```python
from build123d import *

# Parameters (mm, degrees)
BOSS_EXTRUDE1_DEPTH = 5
SKETCH2_W           = 14
SKETCH2_H           = 11.693793348
SKETCH2_W_2         = 9
SKETCH2_H_2         = 16.306206652
SKETCH2_W_3         = 13
SKETCH2_H_3         = 6.693793348
SKETCH2_W_4         = 8
SKETCH2_H_4         = 5
BOSS_EXTRUDE2_DEPTH = 22
BOSS_EXTRUDE3_START = -20
SKETCH3_W           = 12
SKETCH3_H           = 12
BOSS_EXTRUDE3_DEPTH = 7
CUT_EXTRUDE1_START  = -2.25
CUT_EXTRUDE1_DEPTH  = 2.5
SKETCH5_R           = 1.65
CUT_EXTRUDE3_DEPTH  = 28
SKETCH6_W           = 12
SKETCH6_H           = 12
SKETCH6_R           = 1.65
BOSS_EXTRUDE4_DEPTH = 4
BOSS_EXTRUDE6_START = -20
SKETCH7_W           = 12
SKETCH7_H           = 12
SKETCH7_R           = 1.65
BOSS_EXTRUDE6_DEPTH = 7
CUT_EXTRUDE4_START  = -2.25
CUT_EXTRUDE4_DEPTH  = 2.5
SKETCH9_W           = 12
SKETCH9_H           = 12
SKETCH9_R           = 1.65
BOSS_EXTRUDE7_DEPTH = 4


with BuildPart() as part:
    # Sketch1 → Boss-Extrude1 (new body)
    with BuildSketch(Plane(origin=(0, 0, 0), x_dir=(1, 0, 0), z_dir=(0, 1, 0))):
        Polygon((0, 0), (28, 0), (28, 5), (7, 5), (7, 23), (15, 23), (15, 28), (0, 28), align=None)
    extrude(amount=BOSS_EXTRUDE1_DEPTH)

    # Sketch2 → Boss-Extrude2 (add)
    with BuildSketch(Plane(origin=(0, 5, 0), x_dir=(1, 0, 0), z_dir=(0, 1, 0))):
        with Locations((-7, 5.846896674)):
            Rectangle(SKETCH2_W, SKETCH2_H)
        with Locations((-18.5, 5.846896674)):
            Rectangle(SKETCH2_W_2, SKETCH2_H)
        with Locations((-7, 19.846896674)):
            Rectangle(SKETCH2_W, SKETCH2_H_2)
        Polygon((7, 23), (7, 11.693793348), (20, 11.693793348), (20, 28), (15, 28), (15, 23), align=None)
        with Locations((13.5, 8.346896674)):
            Rectangle(SKETCH2_W_3, SKETCH2_H_3)
        Polygon((20, 11.693793348), (20, 5), (28, 5), (28, 0), (30.5, 0), (30.5, 11.693793348), align=None)
        Polygon((0, 11.693793348), (0, 0), (20, 0), (20, 5), (7, 5), (7, 11.693793348), align=None)
        Polygon((0, 28), (0, 11.693793348), (7, 11.693793348), (7, 23), (15, 23), (15, 28), align=None)
        with Locations((24, 2.5)):
            Rectangle(SKETCH2_W_4, SKETCH2_H_4)
    extrude(amount=BOSS_EXTRUDE2_DEPTH)

    # Sketch3 → Boss-Extrude3 (add)
    with BuildSketch(Plane(origin=(0, 27, 0), x_dir=(1, 0, 0), z_dir=(0, 1, 0)).offset(BOSS_EXTRUDE3_START)):
        with Locations((11, 34)):
            Rectangle(SKETCH3_W, SKETCH3_H)
    extrude(amount=-BOSS_EXTRUDE3_DEPTH)

    # Sketch4 → Cut-Extrude1 (cut)
    with BuildSketch(Plane.XZ.offset(CUT_EXTRUDE1_START)):
        Polygon((14.233161507, -36), (12.616580754, -33.2), (9.383419246, -33.2), (7.766838493, -36), (9.383419246, -38.8), (12.616580754, -38.8), align=None)
    extrude(amount=-CUT_EXTRUDE1_DEPTH, mode=Mode.SUBTRACT)

    # Sketch5 → Cut-Extrude3 (cut, through all)
    with BuildSketch(Plane.XZ):
        with Locations((11, -36)):
            Circle(SKETCH5_R)
    extrude(amount=-CUT_EXTRUDE3_DEPTH, mode=Mode.SUBTRACT)

    # Sketch6 → Boss-Extrude4 (add)
    with BuildSketch(Plane(origin=(0, 27, 0), x_dir=(1, 0, 0), z_dir=(0, 1, 0))):
        with Locations((-6, 34)):
            Rectangle(SKETCH6_W, SKETCH6_H)
        with Locations((-6, 34)):
            Circle(SKETCH6_R, mode=Mode.SUBTRACT)
    extrude(amount=-BOSS_EXTRUDE4_DEPTH)

    # Sketch7 → Boss-Extrude6 (add)
    with BuildSketch(Plane(origin=(0, 27, 0), x_dir=(1, 0, 0), z_dir=(0, 1, 0)).offset(BOSS_EXTRUDE6_START)):
        with Locations((6, -6)):
            Rectangle(SKETCH7_W, SKETCH7_H)
        with Locations((6, -8)):
            Circle(SKETCH7_R, mode=Mode.SUBTRACT)
    extrude(amount=-BOSS_EXTRUDE6_DEPTH)

    # Sketch8 → Cut-Extrude4 (cut)
    with BuildSketch(Plane.XZ.offset(CUT_EXTRUDE4_START)):
        Polygon((9.233161507, 8), (7.616580754, 10.8), (4.383419246, 10.8), (2.766838493, 8), (4.383419246, 5.2), (7.616580754, 5.2), align=None)
    extrude(amount=-CUT_EXTRUDE4_DEPTH, mode=Mode.SUBTRACT)

    # Sketch9 → Boss-Extrude7 (add)
    with BuildSketch(Plane(origin=(0, 27, 0), x_dir=(1, 0, 0), z_dir=(0, 1, 0))):
        with Locations((-8, -6)):
            Rectangle(SKETCH9_W, SKETCH9_H)
        with Locations((-8, -6)):
            Circle(SKETCH9_R, mode=Mode.SUBTRACT)
        with Locations((20, -6)):
            Rectangle(SKETCH9_W, SKETCH9_H)
        with Locations((20, -6)):
            Circle(SKETCH9_R, mode=Mode.SUBTRACT)
    extrude(amount=-BOSS_EXTRUDE7_DEPTH)


solid = part.part
```
Build history of the part. All positions in model axes, mm. A direction names the side the tool comes from. Round coordinates to 2 decimals unless told otherwise and drop trailing zeros. Loops run counter-clockwise (first coordinate to the right, second up) from the corner with the lowest first, then second, coordinate; pieces in that order, holes last.
Item 1: Which spindle directions (+Z, -Z, +X, -X, +Y, -Y) get a long thin tool onto all of the face, cutting with end or side? Do faces 1 (the face through (3.564, 3.482, 6.62)), 2 (the face through (21.2, 23, 4.6)), 3 (the face through (-2, 25, 6)). Say none if no direction does.
Item 2: Drill centre lines: line 1 along Z through (x, y) = (11, 1.4); line 2 along X through (y, z) = (26.1, 6); line 3 along X through (y, z) = (5.6, 8). Where is each one in solid material? Low to high.
Item 3: Two-plate mould, pull along Y, no slides. Class faces 4 (the face through (6, 7, 6)), 5 (the face through (20, 16, -20)), 6 (the face through (7.4, 4.75, 9.3)), 7 (the face through (8.414, 3.482, 6.58)): released by +Y, released by -Y, zero draft, split by the parting line, or undercut.
Item 4: Saw through at B-B (x = 6). List the corners of the cut face in (y, z).
Item 5: Saw through at D-D (z = -10.5). List the corners of the cut face in (x, y).
Item 6: Pin check, flat tips, straight feed: P1, Ø6, axis at x = 8, y = 12.5, coming from the +Z side; P2, Ø3, axis at y = 25.5, z = 4, coming from the -X side; P3, Ø13.5, axis at x = -4.5, y = 15.5, coming from the -Z side; P4, Ø1.5, axis at x = -15, z = 3, coming from the -Y side. Stop position of each tip, or through.
Item 7: Saw through at A-A (z = 3). List the corners of the cut face in (x, y).
Item 8: Saw through at C-C (y = 13.5). List the corners of the cut face in (x, z).
Worked answers:
1. face 1: none
1. face 2: +Z, +X, -X, -Y
1. face 3: +Z, +Y, -Y
2. line 1: z = -40 to -37.65, -34.35 to -23, -5 to 12
2. line 2: x = -14 to -9.65, -6.35 to -2, 14 to 18.35, 21.65 to 26
2. line 3: x = 0 to 4.35, 7.65 to 12
3. face 4: released by +Y
3. face 5: zero draft
3. face 6: undercut
3. face 7: undercut
4. outline: (0, -40) - (7, -40) - (7, -28) - (27, -28) - (27, 0) - (7, 0) - (7, 6.35) - (4.75, 6.35) - (4.75, 5.2) - (2.25, 5.2) - (2.25, 6.35) - (0, 6.35) - close; (0, 9.65) - (2.25, 9.65) - (2.25, 10.8) - (4.75, 10.8) - (4.75, 9.65) - (7, 9.65) - (7, 12) - (0, 12) - close
5. outline: (-23, 5) - (0, 5) - (0, 0) - (7, 0) - (7, 5) - (30.5, 5) - (30.5, 27) - (-23, 27) - close
6. P1: stops at z = 0
6. P2: stops at x = -14
6. P3: stops at z = -28
6. P4: passes through
7. outline: (-14, 23) - (-2, 23) - (-2, 27) - (-14, 27) - close; (0, 0) - (12, 0) - (12, 7) - (0, 7) - close; (14, 23) - (26, 23) - (26, 27) - (14, 27) - close
8. outline: (-23, -11.69) - (-14, -11.69) - (-14, -28) - (20, -28) - (20, -11.69) - (30.5, -11.69) - (30.5, 0) - (-23, 0) - close
